Check sheet for the modelled part. Datum: model origin and axes. Units: mm. Face numbers are marked on the shaded views. A direction names the side the tool comes from. Coordinates: 2 decimals unless noted, no trailing zeros. Loops run counter-clockwise (first coordinate to the right, second up) from the corner with the lowest first, then second, coordinate; pieces in that order, holes last. Notation, with made-up numbers: M -18.75,47.25 L 8.25,47.25 A25 ccw 8.25,62.25 Z; hole C 1.5,-37 d8. An arc over 180 degrees is marked long. Write each question's results on one line, items separated by ' | '. Start each with the question number.
from build123d import *

# Parameters (mm, degrees)
F0_R            = 13.49375
F1_DEPTH        = 3.175
F3_DEPTH        = 6.35
F3_COPIES_COUNT = 30
F4_R            = 11.90625
F5_DEPTH        = 1.5875
F6_R            = 11.90625
F7_DEPTH        = 1.5875
F8_R            = 1.5875
F9_DEPTH        = 4.7635
F9_COPIES_COUNT = 4
F10_R           = 3.175
F11_DEPTH       = 1.5875
F12_R           = 3.175
F13_DEPTH       = 1.5875
F14_R           = 1.5875
F15_DEPTH       = 6.351


# Not quite as in the source:
# - a pattern or mirror of a feature is missing from the dataset's text; its kind, count and spacing are read off the source's solid


with BuildPart() as f1:
    # F0 (on Front) → F1 (new body, symmetric)
    with BuildSketch(Plane.XZ):
        Circle(F0_R)
    extrude(amount=F1_DEPTH, both=True)

    # F2 (on face) → F3 (join)
    with BuildSketch(Plane.XZ.offset(3.175)):
        with BuildLine():
            Line((1.7281408885, 16.1722566911), (0.0234068474, 13.4937296987))
            ThreePointArc((0.0234068474, 13.4937296987), (1.4337574514, 13.4173629538), (2.8283995087, 13.1939927725))
            Line((2.8283995087, 13.1939927725), (1.7281408885, 16.1722566911))
        make_face()
    f3 = extrude(amount=-F3_DEPTH)

    # F3_copies: F3 ×30 about axis
    f3_copies_axis = Axis((0, 0, 0), (0, 1, 0))
    for i in range(1, F3_COPIES_COUNT):
        add(f3.rotate(f3_copies_axis, i * 360 / F3_COPIES_COUNT))

    # F4 (on face) → F5 (cut)
    with BuildSketch(Plane.XZ.offset(3.175)):
        Circle(F4_R)
    extrude(amount=-F5_DEPTH, mode=Mode.SUBTRACT)

    # F6 (on face) → F7 (cut)
    with BuildSketch(Plane(origin=(0, 3.175, 0), x_dir=(-1, 0, 0), z_dir=(0, 1, 0))):
        Circle(F6_R)
    extrude(amount=-F7_DEPTH, mode=Mode.SUBTRACT)

    # F8 (on face) → F9 (cut, through all)
    with BuildSketch(Plane.XZ.offset(1.5875)):
        with Locations((-5.6939616362, 5.6939616362)):
            Circle(F8_R)
    f9 = extrude(amount=-F9_DEPTH, mode=Mode.SUBTRACT)

    # F9_copies: F9 ×4 about axis
    f9_copies_axis = Axis((0, 0, 0), (0, 1, 0))
    for i in range(1, F9_COPIES_COUNT):
        add(f9.rotate(f9_copies_axis, i * 360 / F9_COPIES_COUNT), mode=Mode.SUBTRACT)

    # F10 (on face) → F11 (join)
    with BuildSketch(Plane.XZ.offset(1.5875)):
        Circle(F10_R)
    extrude(amount=F11_DEPTH)

    # F12 (on face) → F13 (join)
    with BuildSketch(Plane(origin=(0, 1.5875, 0), x_dir=(-1, 0, 0), z_dir=(0, 1, 0))):
        Circle(F12_R)
    extrude(amount=F13_DEPTH)

    # F14 (on face) → F15 (cut, through all)
    with BuildSketch(Plane(origin=(0, 3.175, 0), x_dir=(-1, 0, 0), z_dir=(0, 1, 0))):
        Circle(F14_R)
    extrude(amount=-F15_DEPTH, mode=Mode.SUBTRACT)


solid = f1.part
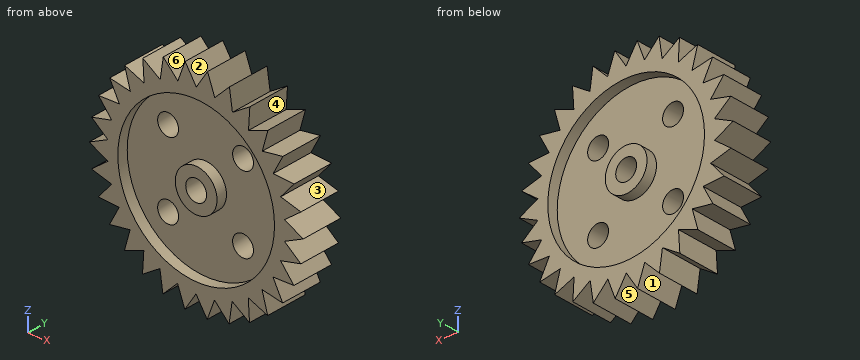
Item 1: Depth check by flat-ended pin: P1, Ø3.5, axis at x = 5.69, z = -5.69, coming from the -Y side; P2, Ø1.9, axis at x = -5.69, z = -5.69, coming from the -Y side; P3, Ø1.5, axis at x = 6.5, y = -1, coming from the +Z side; P4, Ø2, axis at y = -1.5, z = -7.5, coming from the +X side. Enter the tip coordinate at first touch or a pass-through.
Item 2: Section check B-B (z = 1). Record the cut outline in (x, y) (1 decimal).
Item 3: Tool access check on the marked faces 4, 5 and 6. Record the directions out of +Z, -Z, +X, -X, +Y, -Y that give a thin tool (end or side, any length) a straight path to the whole face; none if there is none.
Item 4: Section check D-D (x = -9.5). Record the cut outline in (y, z) (1 decimal), plus the area to 3 significant figures.
Item 5: Section check C-C (z = -8). Record the cut outline in (x, y) (1 decimal).
Item 6: Section check A-A (y = 2.75). State how many separate pieces and enclosed holes the cut face has, plus the area to 3 significant figures.
Item 7: Thickness scan on line 1 (X direction, y = 3, z = 12.5); line 2 (X direction, y = -0.75, z = -5); line 3 (Z direction, x = 12, y = 2.5). Record the ranges inside material, lowest first.
Item 8: Release check for a two-part mould opening along Z. For the marked faces 1, 2 and 3 record: +Z half, -Z half, draft (parallel to the pull), parting line (faces both ways), or undercut.
Computed values:
1) P1: stops at y = -1.59 | P2: passes through | P3: stops at z = 13.47 | P4: stops at x = 14.85
2) outline: M -14.3,-3.2 L -11.9,-3.2 L -11.9,-1.6 L -3,-1.6 L -3,-3.2 L -1.2,-3.2 L -1.2,3.2 L -3,3.2 L -3,1.6 L -11.9,1.6 L -11.9,3.2 L -14.3,3.2 Z; M 1.2,-3.2 L 3,-3.2 L 3,-1.6 L 11.9,-1.6 L 11.9,-3.2 L 14.2,-3.2 L 14.2,3.2 L 11.9,3.2 L 11.9,1.6 L 3,1.6 L 3,3.2 L 1.2,3.2 Z
3) face 4: +Y, -Y | face 5: -Z, +Y, -Y | face 6: +Z, +Y, -Y
4) outline: M -3.2,-11.5 L 3.2,-11.5 L 3.2,-7.2 L 1.6,-7.2 L 1.6,7.2 L 3.2,7.2 L 3.2,11.6 L -3.2,11.6 L -3.2,7.2 L -1.6,7.2 L -1.6,-7.2 L -3.2,-7.2 Z | area: 101 mm²
5) outline: M -12.4,-3.2 L -8.8,-3.2 L -8.8,-1.6 L 8.8,-1.6 L 8.8,-3.2 L 12.3,-3.2 L 12.3,3.2 L 8.8,3.2 L 8.8,1.6 L -8.8,1.6 L -8.8,3.2 L -12.4,3.2 Z
6) separate pieces: 2 | enclosed holes: 2 | area: 267 mm²
7) line 1: x = -8.01 to -5.71, -5.44 to 5.48, 5.79 to 8.05 | line 2: x = -13.55 to -7.12, -4.27 to 4.27, 7.12 to 13.49 | line 3: z = -9.39 to -7.39, -6.75 to 6.71, 7.3 to 9.34
8) face 1: -Z half | face 2: +Z half | face 3: undercut
